Geometry check sheet. Reference: the model listing, model coordinates, mm. A direction names the side the tool comes from. Round coordinates to 2 decimals unless told otherwise and drop trailing zeros. Order: outer loops, then holes, each group sorted by start corner. A loop starts at its lowest first (then second) coordinate and runs counter-clockwise, first axis right, second up. Notation, with made-up numbers: (9.5, 55) -> (38.5, 55) arc R29 ccw to (38.5, 81) -> close; hole circle Ø5 at (83, 3.25). An arc over 180 degrees is marked (long way). Answer as a JSON object with one key per item and string values. Group by question number.
from build123d import *

# Parameters (mm, degrees)
F0_R     = 3.5
F1_DEPTH = 8
F0_W     = 30
F0_H     = 50
F2_DEPTH = 10
F0_W_2   = 20
F3_DEPTH = 12
F4_DEPTH = 14
F0_W_3   = 40
F5_DEPTH = 18
F6_DEPTH = 25


with BuildPart() as f1:
    # F0 (on Front) → F1 (new body)
    with BuildSketch(Plane.XZ):
        Polygon((-70, 100), (-100, 100), (-100, -100), (100, -100), (100, 100), (70, 100), (50, 100), (20, 100), (-20, 100), (-50, 100), align=None)
        with Locations((-70, -70)):
            Circle(F0_R, mode=Mode.SUBTRACT)
        with Locations((70, -70)):
            Circle(F0_R, mode=Mode.SUBTRACT)
        with Locations((-70, 70)):
            Circle(F0_R, mode=Mode.SUBTRACT)
        with Locations((70, 70)):
            Circle(F0_R, mode=Mode.SUBTRACT)
    extrude(amount=F1_DEPTH)

    # F0 (on Front) → F2 (join)
    with BuildSketch(Plane.XZ):
        with Locations((-85, 125)):
            Rectangle(F0_W, F0_H)
        with Locations((85, 125)):
            Rectangle(F0_W, F0_H)
    extrude(amount=F2_DEPTH)

    # F0 (on Front) → F3 (join)
    with BuildSketch(Plane.XZ):
        with Locations((-60, 125)):
            Rectangle(F0_W_2, F0_H)
        with Locations((60, 125)):
            Rectangle(F0_W_2, F0_H)
    extrude(amount=F3_DEPTH)

    # F0 (on Front) → F4 (join)
    with BuildSketch(Plane.XZ):
        with Locations((-35, 125)):
            Rectangle(F0_W, F0_H)
        with Locations((35, 125)):
            Rectangle(F0_W, F0_H)
        Polygon((-50, 200), (-50, 150), (-20, 150), (-20, 200), (-48, 200), align=None)
        Polygon((20, 200), (20, 150), (50, 150), (50, 200), (48, 200), align=None)
    extrude(amount=F4_DEPTH)

    # F0 (on Front) → F5 (join)
    with BuildSketch(Plane.XZ):
        with Locations((0, 125)):
            Rectangle(F0_W_3, F0_H)
        with Locations((0, 175)):
            Rectangle(F0_W_3, F0_H)
    extrude(amount=F5_DEPTH)

    # F0 (on Front) → F6 (join)
    with BuildSketch(Plane.XZ):
        Polygon((-48, 200), (-20, 200), (20, 200), (48, 200), (48, 220), (-48, 220), align=None)
    extrude(amount=F6_DEPTH)


solid = f1.part
Item 1: Sectioned sample at C-C, the plane z = 131. Enter the section's corners in (x, y).
Item 2: Mould release check, pull along Z, two halves, no side actions. Record for faces 1 (the flat face through (-35, -14, 151)), 2 (the flat face through (1, -12, 220)), 3 (the cylindrical face through (-72.58, -3.944, -67.635)): pulls with the +Z half, pulls with the -Z half, needs draft (parallel to the pull), parting line crosses it, or undercut.
Item 3: Thickness scan on L1, parallel to Z at x = -70, y = -1.5; L2, parallel to Z at x = 71.5, y = -3; L3, parallel to Y at x = 59.5, z = 25.5. Record the ranges inside material, lowest first.
Item 4: Sectioned sample at D-D, the plane z = 181. Enter the section's corners in (x, y).
Item 5: Depth check by flat-ended pin: pin 1 Ø16 at (x, z) = (56.5, 124) entering from -Y; pin 2 Ø9.5 at (x, y) = (66.5, -7.5) entering from +Z; pin 3 Ø4 at (y, z) = (-4, 165.5) entering from -X. Enter the tip coordinate at first touch or a pass-through.
Item 6: Set-up check for faces 4 (the flat face through (75, -6, 150)), 5 (the flat face through (-85, -10, 125)), 6 (the flat face through (-1, -8, 1)), 7 (the flat face through (60, -12, 125)), 8 (the cylindrical face through (67.42, -3.944, -67.635)): record each of +Z, -Z, +X, -X, +Y, -Y from which the full face is reachable in a straight line by a thin tool's end or side.
Item 7: Sectioned sample at B-B, the plane x = 24. Enter the section's corners in (y, z).
Item 8: Sectioned sample at A-A, the plane z = 70. Enter the section's corners in (x, y).
Result:
{
 "1": {"outline": "(-100, -10) -> (-70, -10) -> (-70, -12) -> (-50, -12) -> (-50, -14) -> (-20, -14) -> (-20, -18) -> (20, -18) -> (20, -14) -> (50, -14) -> (50, -12) -> (70, -12) -> (70, -10) -> (100, -10) -> (100, 0) -> (-100, 0) -> close"},
 "2": {"face 1": "needs draft", "face 2": "pulls with the +Z half", "face 3": "undercut"},
 "3": {"L1": "z = -100 to -73.5, -66.5 to 66.5, 73.5 to 150", "L2": "z = -100 to -73.16, -66.84 to 66.84, 73.16 to 150", "L3": "y = -8 to 0"},
 "4": {"outline": "(-50, -14) -> (-20, -14) -> (-20, -18) -> (20, -18) -> (20, -14) -> (50, -14) -> (50, 0) -> (-50, 0) -> close"},
 "5": {"pin 1": "stops at y = -14", "pin 2": "stops at z = 150", "pin 3": "stops at x = -50"},
 "6": {"face 4": "+Z, +X, +Y, -Y", "face 5": "+Z, -Z, -X, -Y", "face 6": "-Z, +X, -X, -Y", "face 7": "+Z, -Z, +X, -Y", "face 8": "+Y, -Y"},
 "7": {"outline": "(-25, 200) -> (-14, 200) -> (-14, 100) -> (-8, 100) -> (-8, -100) -> (0, -100) -> (0, 220) -> (-25, 220) -> close"},
 "8": {"outline": "(-100, -8) -> (-73.5, -8) -> (-73.5, 0) -> (-100, 0) -> close; (-66.5, -8) -> (66.5, -8) -> (66.5, 0) -> (-66.5, 0) -> close; (73.5, -8) -> (100, -8) -> (100, 0) -> (73.5, 0) -> close"}
}
